Autodesk Inventor part; units mm, degrees
ref_plane "Plan YZ" through (0, 0, 0) normal (1, 0, 0) x (0, 1, 0)
ref_plane "Plan XZ" through (0, 0, 0) normal (0, 1, 0) x (-1, 0, 0)
ref_plane "Plan XY" through (0, 0, 0) normal (0, 0, 1) x (1, 0, 0)
sketch "Esquisse1" plane through (0, 0, 0) normal (0, 0, 1) x (1, 0, 0)
  line L0 (0, 0) -> (-25, 0)
  line L1 (-25, 0) -> (-25, 8.5)
  line L2 (-25, 8.5) -> (0, 8.5)
  line L3 (0, 8.5) -> (0, 0)
  dimension "d0" = 25
  dimension "d1" = 8.5
extrude "Extrusion1" add sketch "Esquisse1" along normal blind 11.5
sketch "Esquisse6" plane through (0, 0, 11.5) normal (0, 0, 1) x (1, 0, 0)
  line L0 (-18.5, 1.75) -> (-6.5, 1.75)
  line L1 (-6.5, 1.75) -> (-6.5, 6.75)
  line L2 (-6.5, 6.75) -> (-18.5, 6.75)
  line L3 (-18.5, 6.75) -> (-18.5, 1.75)
  line L4 (-6.5, 4.25) -> (0, 4.25) construction
  line L5 (0, 0) -> (0, 8.5)
  line L6 (-25, 4.25) -> (-18.5, 4.25) construction
  line L7 (-25, 8.5) -> (-25, 0) construction
  line L8 (-21.7955, 8.5) -> (-21.7955, 6.75) construction
  line L9 (-18.2379, 0) -> (-18.2379, 1.75) construction
  line L10 (-25, 0) -> (0, 0) construction
  line L11 (0, 8.5) -> (-25, 8.5) construction
  dimension "d4" = 5
  dimension "d5" = 12
extrude "Extrusion2" cut sketch "Esquisse6" against normal blind 1
sketch "Esquisse7" plane through (0, 0, 10.5) normal (0, 0, 1) x (1, 0, 0)
  line L0 (-6.5, 1.75) -> (-12.5, 1.75)
  line L1 (-12.5, 1.75) -> (-12.5, 6.75)
  line L2 (-12.5, 6.75) -> (-6.5, 6.75)
  line L3 (-6.5, 6.75) -> (-6.5, 1.75)
  line L4 (-6.5, 1.75) -> (-18.5, 1.75)
  line L5 (-18.5, 6.75) -> (-6.5, 6.75)
  line L6 (-6.5, 6.75) -> (-6.5, 1.75)
  point P0 (0, 0)
  dimension "d8" = 6
extrude "Extrusion3" add sketch "Esquisse7" along normal blind 7.5
sketch "Esquisse8" plane through (0, 0, 11.5) normal (0, 0, 1) x (1, 0, 0)
  line L0 (-3, 4.354) -> (-3, 0.0702) construction
  line L1 (-3, 8.6378) -> (-3, 4.354) construction
  line L2 (0, 0) -> (0, 8.5) construction
  dimension "d18" = 3
hole "Perçage1" at (-3, 4.354, 11.5) direction (0, 0, -1) diameter 2.013 end through all
sketch "Esquisse9" plane through (0, 0, 11.5) normal (0, 0, 1) x (1, 0, 0)
  line L0 (-25, 8.5) -> (-25, 0)
  line L1 (-22, 0.0375) -> (-22, 4.2687) construction
  line L2 (-22, 4.2687) -> (-22, 8.5) construction
  line L3 (0, 8.5) -> (-25, 8.5) construction
  point P0 (0, 0)
  dimension "d26" = 3
hole "Perçage2" at (-22, 4.2687, 11.5) direction (0, 0, -1) diameter 2.013 end through all
properties part number "P1704_013_Switch" material "."
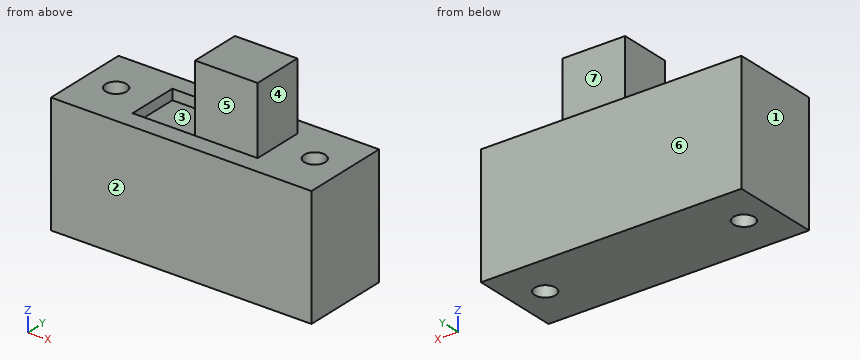
Input: part model. Units: mm. Frame: model coordinates. Face numbers are marked on the shaded views. A direction names the side the tool comes from. Give positions to 0.01 mm unless a question says otherwise; leave off trailing zeros. Write each loop counter-clockwise with the first axis right and the second up, starting at its lowest first coordinate (ties: lowest second). Pieces come first, ordered by that corner, then holes. Notation, with made-up numbers: (36.5, 80.5) - (50.5, 80.5) arc R36 cw to (50.5, 118.5) - close; hole circle Ø1 at (48.25, 59). An arc over 180 degrees is marked (long way). Write item = value, one per line. Start each with the question number.
1. Access query for the marked faces 4, 5, 6 and 7. Directions: +Z, -Z, +X, -X, +Y, -Y. A direction counts if a zero-diameter tool reaches every point of the face in a straight line with its end or side. Return the directions, or none.
2. Section query C-C, the plane z = 3.5. Output: boundary loops of the cut face in (x, y).
3. Mould query, pull axis Y, two halves, no side actions, for the marked faces 1, 2 and 3. Classes: released by +Y, released by -Y, zero draft, split by the parting line, or undercut.
4. Ray query, L1, parallel to Y at x = -22, z = 8.75; L2, parallel to Y at x = -3, z = 3.75; L3, parallel to Z at x = -4.5, y = 2.5. Return the intervals inside material, ascending.
5. First-contact query: pin 1 Ø1.1 at (y, z) = (3.5, 11) entering from +X; pin 2 Ø5 at (x, z) = (-9, 15.5) entering from -Y; pin 3 Ø5 at (x, z) = (-15.5, 16) entering from -Y; pin 4 Ø6 at (x, z) = (-6.5, 15.5) entering from +Y. Flat tips, straight axial feed; report the tip coordinate or a pass-through.
6. Section query A-A, the plane x = -3. Output: boundary loops of the cut face in (y, z).
7. Section query B-B, the plane y = 4. Output: boundary loops of the cut face in (x, z).
8. Section query D-D, the plane y = 6. Output: boundary loops of the cut face in (x, z).
Check sheet entries:
q1.face_4 = +Z, +X, +Y, -Y
q1.face_5 = +Z, +X, -X, -Y
q1.face_6 = +Z, -Z, +X, -X, +Y
q1.face_7 = +Z, +X, -X, +Y
q2.outline = (-25, 0) - (0, 0) - (0, 8.5) - (-25, 8.5) - close; hole circle Ø2.01 at (-22, 4.27); hole circle Ø2.01 at (-3, 4.35)
q3.face_1 = zero draft
q3.face_2 = released by -Y
q3.face_3 = undercut
q4.L1 = 0 to 3.26, 5.28 to 8.5
q4.L2 = 0 to 3.35, 5.36 to 8.5
q4.L3 = 0 to 11.5
q5.pin_1 = 0
q5.pin_2 = 1.75
q5.pin_3 = through
q5.pin_4 = 6.75
q6.outline = (0, 0) - (3.35, 0) - (3.35, 11.5) - (0, 11.5) - close; (5.36, 0) - (8.5, 0) - (8.5, 11.5) - (5.36, 11.5) - close
q7.outline = (-25, 0) - (-22.97, 0) - (-22.97, 11.5) - (-25, 11.5) - close; (-21.03, 0) - (-3.94, 0) - (-3.94, 11.5) - (-6.5, 11.5) - (-6.5, 18) - (-12.5, 18) - (-12.5, 10.5) - (-18.5, 10.5) - (-18.5, 11.5) - (-21.03, 11.5) - close; (-2.06, 0) - (0, 0) - (0, 11.5) - (-2.06, 11.5) - close
q8.outline = (-25, 0) - (0, 0) - (0, 11.5) - (-6.5, 11.5) - (-6.5, 18) - (-12.5, 18) - (-12.5, 10.5) - (-18.5, 10.5) - (-18.5, 11.5) - (-25, 11.5) - close
